Here's the drawing with two shaded views (mm, measured from the low corner). I have some questions. Round coordinates to 2 decimals unless told otherwise and drop trailing zeros. Order: outer loops, then holes, each group sorted by start corner. A loop starts at its lowest first (then second) coordinate and runs counter-clockwise, first axis right, second up. Notation, with made-up numbers: (31, 53.5) -> (69, 53.5) arc R9 ccw to (69, 58.5) -> close; hole circle Ø6 at (38.25, 49). An arc over 180 degrees is marked (long way). Use a Markdown table: item, result. Add a question column.
Q1. I'm going to push flat-ended pins straight in: pin 1 Ø1.5 at (x, y) = (22, 1) entering from +Z; pin 2 Ø1.5 at (x, y) = (58, 4) entering from +Z. Where does each tip first touch, or does it pass through?
Q2. I need wall thicknesses on line 1 along Z through (x, y) = (38, 0.8); line 2 along X through (y, z) = (2, 38). Which ranges of each line are inside material? Lowest first, please. Write a range as [from, to].
Q3. We'd pull the mould along Z, two halves only. Please class the marked faces 1 and 2: +Z half, -Z half, draft (parallel to the pull), parting line (faces both ways), or undercut.
Q4. If we section it at C-C on y = 2.25: List the corners of the cut face in (x, z) for me, plus the area to 3 significant figures.
Q5. If we section it at B-B on x = 38: List the corners of the cut face in (y, z) for me, plus the area to 3 significant figures.
Q6. If we section it at A-A on z = 38: List the corners of the cut face in (x, y) for me.
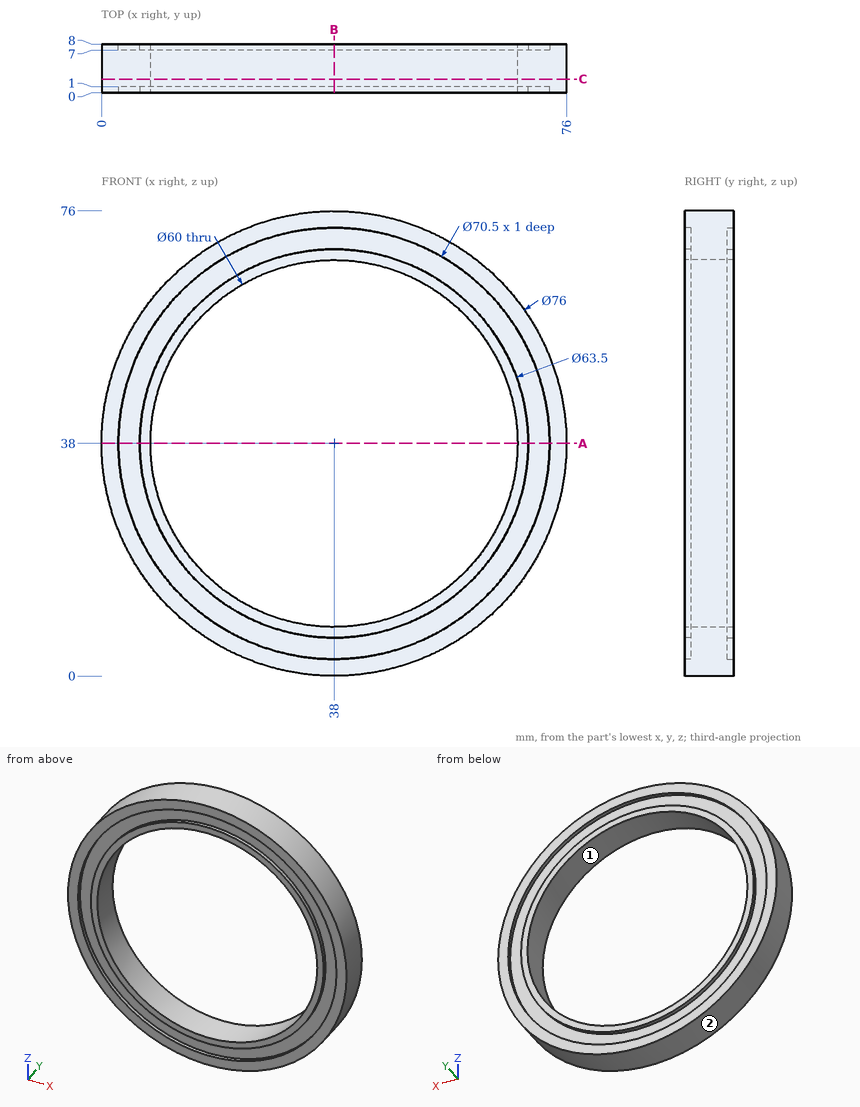
Answer below:
| question | item | result |
|---|---|---|
| 1 | pin 1 | z = 72.81 |
| 1 | pin 2 | z = 70.76 |
| 2 | line 1 | [0, 2.75], [6.25, 8], [68, 69.75], [73.25, 76] |
| 2 | line 2 | [0, 8], [68, 76] |
| 3 | face 1 | undercut |
| 3 | face 2 | parting line |
| 4 | outline | circle Ø76 at (38, 38); hole circle Ø60 at (38, 38) |
| 4 | area | 1,710 mm² |
| 5 | outline | (0, 0) -> (8, 0) -> (8, 2.75) -> (7, 2.75) -> (7, 6.25) -> (8, 6.25) -> (8, 8) -> (0, 8) -> (0, 6.25) -> (1, 6.25) -> (1, 2.75) -> (0, 2.75) -> close; (0, 68) -> (8, 68) -> (8, 69.75) -> (7, 69.75) -> (7, 73.25) -> (8, 73.25) -> (8, 76) -> (0, 76) -> (0, 73.25) -> (1, 73.25) -> (1, 69.75) -> (0, 69.75) -> close |
| 5 | area | 114 mm² |
| 6 | outline | (0, 0) -> (2.75, 0) -> (2.75, 1) -> (6.25, 1) -> (6.25, 0) -> (8, 0) -> (8, 8) -> (6.25, 8) -> (6.25, 7) -> (2.75, 7) -> (2.75, 8) -> (0, 8) -> close; (68, 0) -> (69.75, 0) -> (69.75, 1) -> (73.25, 1) -> (73.25, 0) -> (76, 0) -> (76, 8) -> (73.25, 8) -> (73.25, 7) -> (69.75, 7) -> (69.75, 8) -> (68, 8) -> close |
